Geometry: final body of the model. Coordinates: model frame, mm. Face numbers are marked on the shaded views. A direction names the side the tool comes from. Round coordinates to 2 decimals unless told otherwise and drop trailing zeros. Loops run counter-clockwise (first coordinate to the right, second up) from the corner with the lowest first, then second, coordinate; pieces in that order, holes last. Notation, with made-up numbers: (6.25, 34.25) -> (12.25, 34.25) arc R23 cw to (12.25, 50.25) -> close; hole circle Ø7 at (-14.75, -23.5). An arc over 180 degrees is marked (long way). Answer in a Markdown table with one row per item.
```python
from build123d import *

# Parameters (mm, degrees)
SKETCH1_W           = 170
SKETCH1_H           = 170
BOSS_EXTRUDE1_DEPTH = 1.8
FILLET1_R           = 2
SKETCH2_R           = 1.98
CUT_EXTRUDE1_DEPTH  = 2
SKETCH3_W           = 16
SKETCH3_H           = 20
SKETCH3_W_2         = 37.5
SKETCH3_H_2         = 16.121954722
SKETCH3_W_3         = 18
SKETCH3_H_3         = 16.061076517
SKETCH3_W_4         = 19
SKETCH3_H_4         = 16.780154479
SKETCH3_H_5         = 20.801567196
SKETCH3_W_5         = 25
SKETCH3_H_6         = 17.641885776
BOSS_EXTRUDE2_DEPTH = 35
SKETCH4_W           = 140
SKETCH4_H           = 7
BOSS_EXTRUDE3_DEPTH = 35
LPATTERN1_COUNT     = 2
LPATTERN1_PITCH     = 8
SKETCH5_R           = 45
SKETCH5_R_2         = 39
BOSS_EXTRUDE4_DEPTH = 36


with BuildPart() as part:
    # Sketch1 → Boss-Extrude1 (new body)
    with BuildSketch(Plane(origin=(0, 0, 0), x_dir=(1, 0, 0), z_dir=(0, 1, 0))):
        Rectangle(SKETCH1_W, SKETCH1_H)
    extrude(amount=BOSS_EXTRUDE1_DEPTH)

    # Fillet1
    fillet1_edges = [part.edges().sort_by_distance(p)[0] for p in [
        (-85, 0.9, -85),
        (85, 0.9, -85),
        (85, 0.9, 85),
        (-85, 0.9, 85),
    ]]
    fillet(fillet1_edges, radius=FILLET1_R)

    # Sketch2 → Cut-Extrude1 (cut)
    with BuildSketch(Plane(origin=(0, 1.8, 0), x_dir=(1, 0, 0), z_dir=(0, 1, 0))):
        with Locations((-78.65, 74.84)):
            Circle(SKETCH2_R)
        with Locations((-78.65, -80.1)):
            Circle(SKETCH2_R)
        with Locations((78.83, -80.1)):
            Circle(SKETCH2_R)
        with Locations((78.83, 51.98)):
            Circle(SKETCH2_R)
    extrude(amount=-CUT_EXTRUDE1_DEPTH, mode=Mode.SUBTRACT)

    # Sketch3 → Boss-Extrude2 (add)
    with BuildSketch(Plane(origin=(0, 1.8, 0), x_dir=(1, 0, 0), z_dir=(0, 1, 0))):
        with Locations((74, 75)):
            Rectangle(SKETCH3_W, SKETCH3_H)
        with Locations((16.25, 83.939022639)):
            Rectangle(SKETCH3_W_2, SKETCH3_H_2)
        with Locations((48, 76.969461741)):
            Rectangle(SKETCH3_W_3, SKETCH3_H_3)
        with Locations((-15.17206747, 76.609922761)):
            Rectangle(SKETCH3_W_4, SKETCH3_H_4)
        with Locations((-34.244584998, 74.599216402)):
            Rectangle(SKETCH3_W, SKETCH3_H_5)
        with Locations((-56.603208404, 76.179057112)):
            Rectangle(SKETCH3_W_5, SKETCH3_H_6)
    extrude(amount=BOSS_EXTRUDE2_DEPTH)

    # Sketch4 → Boss-Extrude3 (add)
    with BuildSketch(Plane(origin=(0, 1.8, 0), x_dir=(1, 0, 0), z_dir=(0, 1, 0))):
        with Locations((9, -68.5)):
            Rectangle(SKETCH4_W, SKETCH4_H)
    boss_extrude3 = extrude(amount=BOSS_EXTRUDE3_DEPTH)

    # LPattern1: Boss-Extrude3 ×2
    with Locations(*[(0, 0, -i * LPATTERN1_PITCH) for i in range(1, LPATTERN1_COUNT)]):
        add(boss_extrude3)

    # Sketch5 → Boss-Extrude4 (add)
    with BuildSketch(Plane(origin=(0, 1.8, 0), x_dir=(1, 0, 0), z_dir=(0, 1, 0))):
        with Locations((-25, -9)):
            Circle(SKETCH5_R)
        with Locations((-25, -9)):
            Circle(SKETCH5_R_2, mode=Mode.SUBTRACT)
    extrude(amount=BOSS_EXTRUDE4_DEPTH)


solid = part.part
```
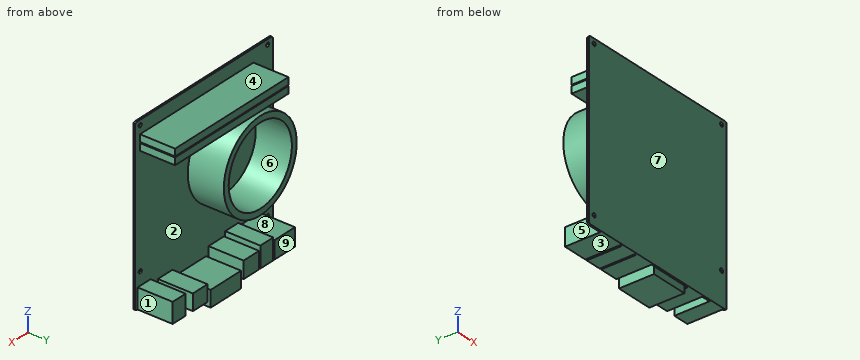
Item 1: Section query A-A, the plane y = 13.5. State how many separate pieces and enclosed holes the cut face has, and give its area (3 significant figures).
Ans:
| item | result |
|---|---|
| separate pieces | 9 |
| enclosed holes | 1 |
| area | 5,850 mm2 |
Item 2: First-contact query: P1, Ø3, axis at x = -42.5, y = 25, coming from the -Z side; P2, Ø6, axis at y = 30.5, z = 56.5, coming from the -X side; P3, Ø13, axis at x = 75.5, z = -79.5, coming from the +Y side. Flat tips, straight axial feed; report the tip coordinate or a pass-through.
Ans:
| item | result |
|---|---|
| P1 | z = -85 |
| P2 | x = -61 |
| P3 | y = 36.8 |
Item 3: Section query C-C, the plane z = 9. Output: boundary loops of the cut face in (x, y), and give its area (3 significant figures).
Ans:
| item | result |
|---|---|
| outline | (-85, 0) -> (85, 0) -> (85, 1.8) -> (20, 1.8) -> (20, 37.8) -> (14, 37.8) -> (14, 1.8) -> (-64, 1.8) -> (-64, 37.8) -> (-70, 37.8) -> (-70, 1.8) -> (-85, 1.8) -> close |
| area | 738 mm2 |
Item 4: Set-up query: the marked faces 5, 6, 7, 8 and 9. Return all of +Z, -Z, +X, -X, +Y, -Y with unobstructed straight access to the full face (end or side cutting, diameter ignored); none if empty.
Ans:
| item | result |
|---|---|
| face 5 | -Z, -X, +Y |
| face 6 | +Y |
| face 7 | +Z, -Z, +X, -X, -Y |
| face 8 | -X, +Y |
| face 9 | -Z, +X, -X, +Y |
Item 5: Mould query, pull axis Z, two halves, no side actions, for the marked faces 1, 2, 3 and 4. Classes: released by +Z, released by -Z, zero draft, split by the parting line, or undercut.
Ans:
| item | result |
|---|---|
| face 1 | zero draft |
| face 2 | undercut |
| face 3 | released by -Z |
| face 4 | released by +Z |
Item 6: Ray query, L1, parallel to X at y = 36, z = -68; L2, parallel to Z at x = 31, y = 31; L3, parallel to Z at x = 78.83, y = 1.05. Return the intervals inside material, ascending.
Ans:
| item | result |
|---|---|
| L1 | -69.1 to -44.1, -42.24 to -26.24, 66 to 82 |
| L2 | -92 to -75.88, 57 to 64, 65 to 72 |
| L3 | -85 to -53.96, -50 to 78.12, 82.08 to 85 |
Item 7: Section query D-D, the plane x = -30.5. Output: boundary loops of the cut face in (y, z).
Ans:
| item | result |
|---|---|
| outline | (0, -85) -> (36.8, -85) -> (36.8, -64.2) -> (1.8, -64.2) -> (1.8, -35.66) -> (37.8, -35.66) -> (37.8, -29.61) -> (1.8, -29.61) -> (1.8, 47.61) -> (37.8, 47.61) -> (37.8, 53.66) -> (1.8, 53.66) -> (1.8, 57) -> (36.8, 57) -> (36.8, 64) -> (1.8, 64) -> (1.8, 65) -> (36.8, 65) -> (36.8, 72) -> (1.8, 72) -> (1.8, 85) -> (0, 85) -> close |
Item 8: Section query B-B, the plane x = 71.5. Output: boundary loops of the cut face in (y, z).
Ans:
| item | result |
|---|---|
| outline | (0, -85) -> (36.8, -85) -> (36.8, -65) -> (1.8, -65) -> (1.8, 57) -> (36.8, 57) -> (36.8, 64) -> (1.8, 64) -> (1.8, 65) -> (36.8, 65) -> (36.8, 72) -> (1.8, 72) -> (1.8, 85) -> (0, 85) -> close |
